For this review, use the dimensioned drawing (mm, ordinates from the lowest corner) and the shaded views. A direction names the side the tool comes from. Coordinates: 2 decimals unless noted, no trailing zeros. Loops run counter-clockwise (first coordinate to the right, second up) from the corner with the lowest first, then second, coordinate; pieces in that order, holes last. Notation, with made-up numbers: M -13.75,24 L 35.25,24 A15 cw 35.25,49 Z; hole C 17.25,86.25 d8. An arc over 180 degrees is marked long. Write item = value, one per line. Start each with the question number.
Q1. We need section D-D on z = 27.5. Give the boundary of the cut face in (x, y), and give its area (3 significant figures).
Q2. For the marked faces 1 and 2, list the 3-axis set-ups (+Z, -Z, +X, -X, +Y, -Y) from which the entire face can be reached by the end or side of a thin tool; tool diameter is ignored.
Q3. Wall thickness on probe 1 along Y at (x, z) = (33, 0.6); probe 2 along Y at (x, z) = (5, 6); probe 3 along Z at (x, y) = (12.5, 17.5): over which ranges is each line inside the solid? List them lowest first.
Q4. We need section C-C on z = 20. Give the boundary of the cut face in (x, y).
Q5. We need section B-B on y = 22.5. Give the boundary of the cut face in (x, z).
Q6. We need section A-A on x = 8. Give the boundary of the cut face in (y, z).
Q7. Clearance check with flat-ended pins moving along their axes: pin 1 Ø3 at (x, y) = (33, 32.23) entering from +Z; pin 2 Ø4.5 at (x, y) = (33, 6.23) entering from +Z; pin 3 Ø2 at (x, y) = (13.5, 31) entering from +Z. State where each tip first meets the part, or that it passes through.
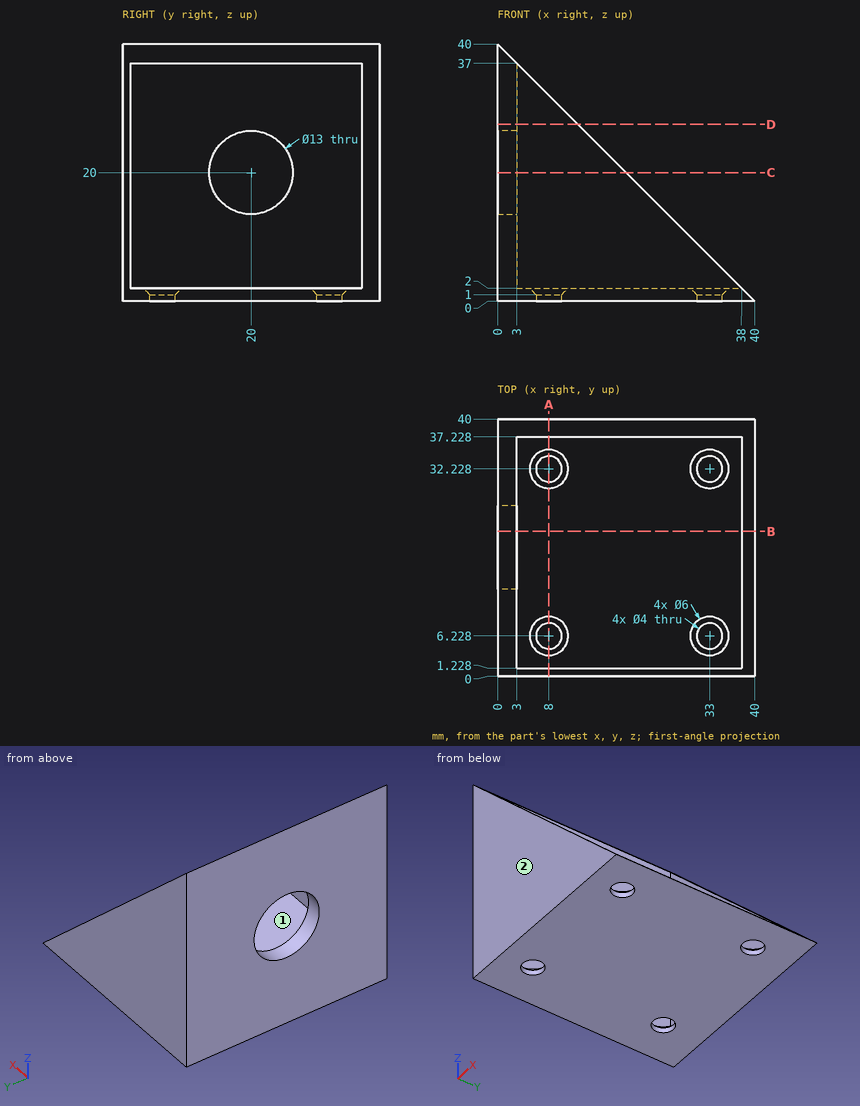
Returned:
q1.outline = M 0,0 L 12.5,0 L 12.5,1.23 L 3,1.23 L 3,37.23 L 12.5,37.23 L 12.5,40 L 0,40 Z
q1.area = 158 mm^2
q2.face_1 = +Z, +X
q2.face_2 = +Z, -Z, +X, -X, -Y
q3.probe_1 = 0 to 4.23, 8.23 to 30.23, 34.23 to 40
q3.probe_2 = 0 to 1.23, 37.23 to 40
q3.probe_3 = 0 to 2
q4.outline = M 0,0 L 20,0 L 20,1.23 L 3,1.23 L 3,13.5 L 0,13.5 Z; M 0,26.5 L 3,26.5 L 3,37.23 L 20,37.23 L 20,40 L 0,40 Z
q5.outline = M 0,0 L 40,0 L 38,2 L 3,2 L 3,14 L 0,14 Z; M 0,26 L 3,26 L 3,37 L 0,40 Z
q6.outline = M 0,0 L 4.23,0 L 4.23,1 L 3.23,2 L 1.23,2 L 1.23,32 L 0,32 Z; M 8.23,0 L 30.23,0 L 30.23,1 L 29.23,2 L 9.23,2 L 8.23,1 Z; M 34.23,0 L 40,0 L 40,32 L 37.23,32 L 37.23,2 L 35.23,2 L 34.23,1 Z
q7.pin_1 = through
q7.pin_2 = 1.25
q7.pin_3 = 2
